The listing builds one solid part. Answer for the finished solid, in the listing's coordinates (mm). A direction names the side the tool comes from. Coordinates: 2 decimals unless noted, no trailing zeros. Write each loop counter-clockwise with the first axis right and the second up, starting at its lowest first coordinate (ties: lowest second). Pieces come first, ordered by that corner, then holes.
from build123d import *

# Parameters (mm, degrees)
SKETCH1_W           = 8.89
SKETCH1_H           = 6.86
EXTRUDE1_DEPTH      = 6.35
SKETCH2_R           = 3.43
EXTRUDE2_DEPTH      = 8.89
SKETCH4_R           = 2.5
EXTRUDE3_DEPTH      = 0.5
SKETCH5_W           = 0.76
SKETCH5_H           = 2.03
EXTRUDE4_DEPTH      = 3.94
LPATTERN1_COUNT     = 3
LPATTERN1_PITCH     = 4.7
CUT_EXTRUDE1_DEPTH  = 23.912952669
BOSS_EXTRUDE1_DEPTH = 1.651
SKETCH8_W           = 0.508
SKETCH8_H           = 5.08
BOSS_EXTRUDE2_DEPTH = 1.651


with BuildPart() as part:
    # Sketch1 → Extrude1 (new, symmetric)
    with BuildSketch(Plane.XY):
        with Locations((4.445, 0)):
            Rectangle(SKETCH1_W, SKETCH1_H)
    extrude(amount=EXTRUDE1_DEPTH, both=True)

    # Sketch2 → Extrude2 (add)
    with BuildSketch(Plane.ZY):
        with Locations(Location((0, 0, 0), (0, 0, 270))):
            Circle(SKETCH2_R)
    extrude(amount=EXTRUDE2_DEPTH)

    # Sketch4 → Extrude3 (cut)
    with BuildSketch(Plane.ZY.offset(8.89)):
        Circle(SKETCH4_R)
    extrude(amount=-EXTRUDE3_DEPTH, mode=Mode.SUBTRACT)

    # Sketch3 → Revolve3 (revolve)
    with BuildSketch(Plane(origin=(0, 0, 0), x_dir=(1, 0, 0), z_dir=(0, 1, 0))):
        with BuildLine():
            Line((-6.5, 0.5), (-5.882977338, -0.823209369))
            Line((-5.882977338, -0.823209369), (-17.482977338, -6.232378204))
            ThreePointArc((-17.482977338, -6.232378204), (-18.599349409, -6.281120061), (-19.423209369, -5.526191497))
            Line((-19.423209369, -5.526191497), (-6.5, 0.5))
        make_face()
    revolve(axis=Axis((-8.89, 0, 0.614475303), (-0.9063077870366493, 0, 0.4226182617407009)))

    # Sketch5 → Extrude4 (add)
    with BuildSketch(Plane(origin=(8.89, 0, 0), x_dir=(0, 0, -1), z_dir=(1, 0, 0))):
        with Locations((-4.7, 0)):
            Rectangle(SKETCH5_W, SKETCH5_H)
    extrude4 = extrude(amount=EXTRUDE4_DEPTH)

    # LPattern1: Extrude4 ×3
    with Locations(*[(0, 0, -i * LPATTERN1_PITCH) for i in range(1, LPATTERN1_COUNT)]):
        add(extrude4)

    # Sketch6 → Cut-Extrude1 (cut, through all)
    with BuildSketch(Plane.XY.offset(5.08)):
        with BuildLine():
            Line((12.205788302, 0.5578), (10.634811698, 0.5578))
            ThreePointArc((10.634811698, 0.5578), (10.4678, 0), (10.634811698, -0.5578))
            Line((10.634811698, -0.5578), (12.205788302, -0.5578))
            ThreePointArc((12.205788302, -0.5578), (12.3728, 0), (12.205788302, 0.5578))
        make_face()
    extrude(amount=-CUT_EXTRUDE1_DEPTH, mode=Mode.SUBTRACT)

    # Sketch7 → Boss-Extrude1 (add)
    with BuildSketch(Plane.ZY):
        Polygon((-4.443403142, 0), (-2.221701571, -3.8481), (2.221701571, -3.8481), (4.443403142, 0), (2.221701571, 3.8481), (-2.221701571, 3.8481), align=None)
    extrude(amount=BOSS_EXTRUDE1_DEPTH)

    # Sketch8 → Revolve4 (revolve)
    with BuildSketch(Plane(origin=(0, 0, 0), x_dir=(1, 0, 0), z_dir=(0, 1, 0)), mode=Mode.PRIVATE) as revolve4_sk:
        with Locations((-3.048, -2.54)):
            Rectangle(SKETCH8_W, SKETCH8_H)
    revolve(revolve4_sk.sketch.rotate(Axis((-2.794, 0, 0), (-1, 0, 0)), 180), axis=Axis((-2.794, 0, 0), (-1, 0, 0)))

    # Sketch9 → Boss-Extrude2 (add)
    with BuildSketch(Plane.ZY.offset(3.302)):
        Polygon((0, 4.443403142), (-3.8481, 2.221701571), (-3.8481, -2.221701571), (0, -4.443403142), (3.8481, -2.221701571), (3.8481, 2.221701571), align=None)
    extrude(amount=BOSS_EXTRUDE2_DEPTH)


solid = part.part
1. A tool of negligible diameter and unlimited length cuts with its end or side. For faces 1 (the cylindrical face through (-8.64, -2.44, -0.54)), 2 (the flat face through (-4.116, 3.348, -1.897)), 3 (the flat face through (4, -3.43, 0)), 4 (the flat face through (-4.116, -3.317, -1.951)), from which of +Z, -Z, +X, -X, +Y, -Y can it reach the whole face along a straight path? Write none if from no direction.
Results found:
face 1: none
face 2: -Z, -X, +Y
face 3: +Z, -Z, +X, -Y
face 4: -Z, -X, -Y
2. Flat-ended cylindrical pins translate along their axes: P1, Ø5, axis at y = 0.5, z = 2, coming from the -X side; P2, Ø0.5, axis at x = -0.5, z = -1, coming from the +Y side; P3, Ø2, axis at x = 3, z = -1.5, coming from the +Y side. Find the tip coordinate at first contact, or state that the pin passes through.
Results found:
P1: stops at x = -19.49
P2: stops at y = 3.85
P3: stops at y = 3.43
3. Section C-C on x = -7.5 is taken. Give the vertices of the cut face in (y, z).
Results found:
outline: circle Ø6.86 at (0, 0)
4. Find the intervals of material crossed by L1, parallel to Y at x = -8.6, z = 0; L2, parallel to X at y = 3.5, z = -0.75; L3, parallel to X at y = 1.5, z = 4, in increasing order.
Results found:
L1: y = -3.43 to -2.5, -1.39 to 1.39, 2.5 to 3.43
L2: x = -4.95 to -2.79, -1.65 to 0
L3: x = -3.3 to -2.79, 0 to 8.89
5. Section A-A on x = -1 is taken. Give the vertices of the cut face in (y, z).
Results found:
outline: (-3.85, -2.22) - (0, -4.44) - (3.85, -2.22) - (3.85, 2.22) - (0, 4.44) - (-3.85, 2.22) - close
6. Section B-B on y = 3 is taken. Give the vertices of the cut face in (x, z), then the cut area to 3 significant figures.
Results found:
outline: (-8.89, -1.66) - (-4.95, -1.66) - (-4.95, -2.5) - (-3.3, -2.5) - (-3.3, -4.1) - (-2.79, -4.1) - (-2.79, -1.66) - (-1.65, -1.66) - (-1.65, -2.71) - (0, -2.71) - (0, -6.35) - (8.89, -6.35) - (8.89, 6.35) - (0, 6.35) - (0, 2.71) - (-1.65, 2.71) - (-1.65, 1.66) - (-2.79, 1.66) - (-2.79, 4.1) - (-3.3, 4.1) - (-3.3, 2.5) - (-4.95, 2.5) - (-4.95, 1.66) - (-8.89, 1.66) - close
area: 151 mm2
7. For a pull along Z with two mould halves and no side action, classify faces 5 (the flat face through (10, 0, -0.38)), 6 (the flat face through (4, 3.43, 0)), 7 (the cylindrical face through (-3.044, -5.037, 0.661)) as pulls with the +Z half, pulls with the -Z half, needs draft (parallel to the pull), parting line crosses it, or undercut.
Results found:
face 5: undercut
face 6: needs draft
face 7: parting line crosses it
